```python
from build123d import *

# Parameters (mm, degrees)
SKETCH1_R           = 47.625
BOSS_EXTRUDE1_DEPTH = 3.175
SKETCH2_R           = 3.175
CUT_EXTRUDE1_DEPTH  = 263.398
SKETCH3_R           = 3.175
CUT_EXTRUDE2_DEPTH  = 25.4
SKETCH4_R           = 1.5875
SKETCH4_R_2         = 1.25
CUT_EXTRUDE3_DEPTH  = 50.8


with BuildPart() as part:
    # Sketch1 → Boss-Extrude1 (new body)
    with BuildSketch(Plane(origin=(0, 0, 0), x_dir=(1, 0, 0), z_dir=(0, 1, 0))):
        with Locations(Location((0, 0, 0), (0, 0, 270))):
            Circle(SKETCH1_R)
    extrude(amount=BOSS_EXTRUDE1_DEPTH)

    # Sketch2 → Cut-Extrude1 (cut)
    with BuildSketch(Plane(origin=(-55.039702575, 231.775, -116.088398355), x_dir=(-1, 0, 0), z_dir=(0, 1, 0))):
        with Locations(Location((-93.139702575, 116.088398355, 0), (0, 0, 90))):
            Circle(SKETCH2_R)
        with Locations(Location((-16.939702575, 116.088398355, 0), (0, 0, 90))):
            Circle(SKETCH2_R)
    extrude(amount=-CUT_EXTRUDE1_DEPTH, mode=Mode.SUBTRACT)

    # Sketch3 → Cut-Extrude2 (cut)
    with BuildSketch(Plane(origin=(-28.264398128, -3.175, -82.371298873), x_dir=(1, 0, 0), z_dir=(0, -1, 0))):
        with Locations(Location((28.264398128, 98.246298873, 0), (0, 0, 90))):
            Circle(SKETCH3_R)
        with Locations(Location((28.264398128, 66.496298873, 0), (0, 0, 90))):
            Circle(SKETCH3_R)
    extrude(amount=-CUT_EXTRUDE2_DEPTH, mode=Mode.SUBTRACT)

    # Sketch4 → Cut-Extrude3 (cut)
    with BuildSketch(Plane(origin=(-28.264398128, -3.175, -82.371298873), x_dir=(-1, 0, 0), z_dir=(0, -1, 0))):
        with Locations(Location((-3.404148128, -108.914298873, 0), (0, 0, 270))):
            Circle(SKETCH4_R)
        with Locations(Location((-12.802148128, -108.914298873, 0), (0, 0, 270))):
            Circle(SKETCH4_R)
        with Locations(Location((-43.726648128, -108.914298873, 0), (0, 0, 270))):
            Circle(SKETCH4_R)
        with Locations(Location((-53.124648128, -108.914298873, 0), (0, 0, 270))):
            Circle(SKETCH4_R)
        with Locations(Location((-8.103148128, -97.230298873, 0), (0, 0, 270))):
            Circle(SKETCH4_R_2)
        with Locations(Location((-48.425648128, -97.230298873, 0), (0, 0, 270))):
            Circle(SKETCH4_R_2)
    extrude(amount=-CUT_EXTRUDE3_DEPTH, mode=Mode.SUBTRACT)


solid = part.part
```
The model under review builds one solid part; all positions refer to its coordinate system, in mm. Coordinates: 2 decimals unless noted, no trailing zeros. Write each loop counter-clockwise with the first axis right and the second up, starting at its lowest first coordinate (ties: lowest second). Pieces come first, ordered by that corner, then holes.
1) We need section C-C on x = -38.1. State the section outline as (y, z) points (3 decimals), then the cut area to 3 significant figures.
2) Clearance check with flat-ended pins moving along their axes: pin 1 Ø1.5 at (y, z) = (1, -19) entering from -X; pin 2 Ø2 at (x, z) = (20.16, 14.86) entering from +Y. State where each tip first meets the part, or that it passes through.
3) We need section D-D on z = -37. State the section outline as (x, y) points (3 decimals), then the cut area to 3 significant figures.
4) To check wall thickness, follow probe 1 along X at (y, z) = (0.7, 0) (3 decimals); probe 2 along Z at (x, y) = (-0.5, 0.7); probe 3 along Z at (x, y) = (-26, 2.8). State the ranges of each line that lie inside material, in increasing order.
5) The part is to be moulded in two halves that separate along Z. For faces 1 (the face through (24.383, 1.565, 28.057)), 2 (the face through (-46.492, 1.565, -10.324)), 3 (the face through (1, 0, -1)), 4 (the face through (-0.954, 1.565, 18.903)), say which applies: pulls with the +Z half, pulls with the -Z half, needs draft (parallel to the pull), parting line crosses it, or undercut.
6) We need section A-A on x = 0. State the section outline as (y, z) points (3 decimals).
7) We need section B-B on y = 1.45. Count the separate pieces of the cut face and the enclosed holes in it, then the cut area to 3 significant figures.
Answer list:
1. outline: (0, -28.575) - (3.175, -28.575) - (3.175, -3.175) - (0, -3.175) - close; (0, 3.175) - (3.175, 3.175) - (3.175, 28.575) - (0, 28.575) - close
1. area: 161 mm2
2. pin 1: stops at x = -43.99
2. pin 2: passes through
3. outline: (-29.986, 0) - (29.986, 0) - (29.986, 3.175) - (-29.986, 3.175) - close
3. area: 190 mm2
4. probe 1: x = -47.625 to -41.275, -34.925 to 34.925, 41.275 to 47.625
4. probe 2: z = -47.62 to -19.01, -12.74 to 12.74, 19.01 to 47.62
4. probe 3: z = -39.9 to 25.44, 27.65 to 39.9
5. face 1: undercut
5. face 2: parting line crosses it
5. face 3: needs draft
5. face 4: undercut
6. outline: (0, -47.625) - (3.175, -47.625) - (3.175, -19.05) - (0, -19.05) - close; (0, -12.7) - (3.175, -12.7) - (3.175, 12.7) - (0, 12.7) - close; (0, 19.05) - (3.175, 19.05) - (3.175, 47.625) - (0, 47.625) - close
7. separate pieces: 1
7. enclosed holes: 10
7. area: 6,960 mm2
